The figure shows three views and two pictorial views of one solid part (mm, origin at its lowest corner). Answer the questions. Coordinates: 2 decimals unless noted, no trailing zeros. Write each loop counter-clockwise with the first axis right and the second up, starting at its lowest first coordinate (ties: lowest second). Pieces come first, ordered by that corner, then holes.
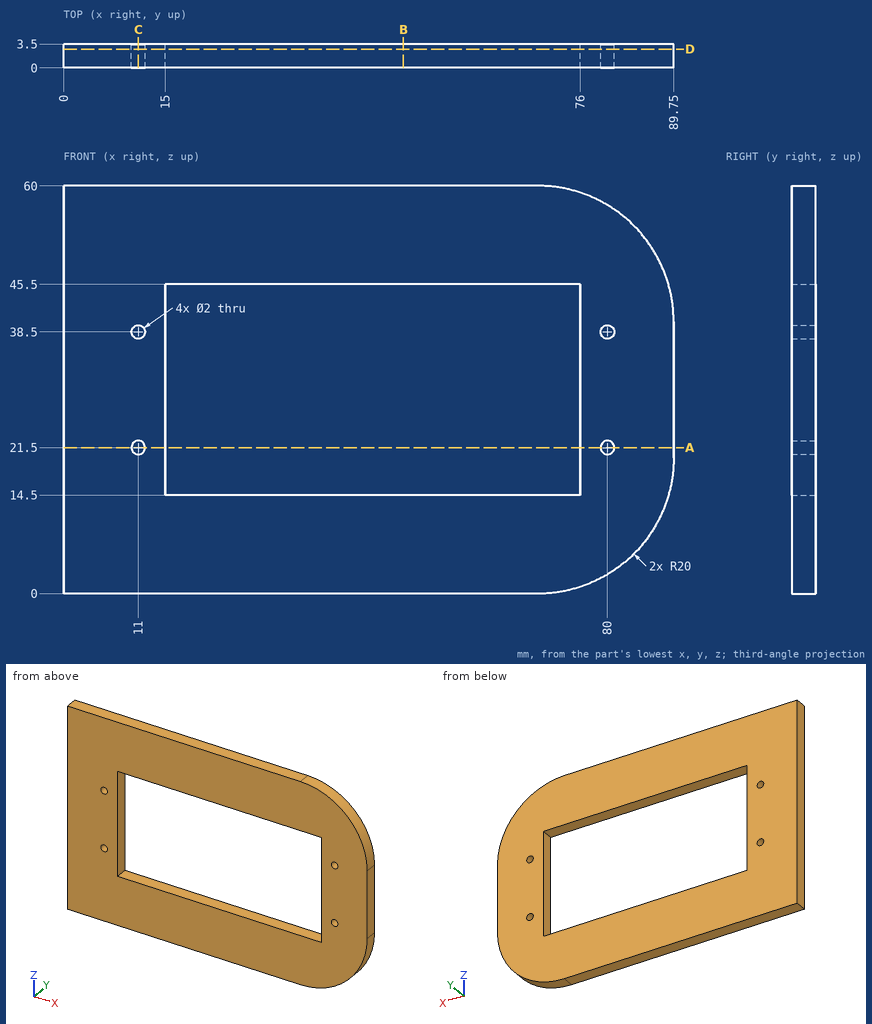
Q1. Find the intervals of material crossed by probe 1 along X at (y, z) = (1, 38.5); probe 2 along Z at (x, y) = (11, 1.35); probe 3 along Z at (x, y) = (51.5, 0.25), in increasing order.
Answers below:
probe 1: x = 0 to 10, 12 to 15, 76 to 79, 81 to 89.75
probe 2: z = 0 to 20.5, 22.5 to 37.5, 39.5 to 60
probe 3: z = 0 to 14.5, 45.5 to 60
Q2. The part is cut by section B-B, the plane x = 50. Write down the section's boundary in (y, z), then the cut area to 4 significant figures.
Answers below:
outline: (0, 0) - (3.5, 0) - (3.5, 14.5) - (0, 14.5) - close; (0, 45.5) - (3.5, 45.5) - (3.5, 60) - (0, 60) - close
area: 101.5 mm2
Q3. The part is cut by section D-D, the plane y = 2.75. Write down the section's boundary in (x, z).
Answers below:
outline: (0, 0) - (69.75, 0) arc R20 ccw to (89.75, 20) - (89.75, 40) arc R20 ccw to (69.75, 60) - (0, 60) - close; hole circle Ø2 at (11, 21.5); hole circle Ø2 at (11, 38.5); hole (15, 14.5) - (76, 14.5) - (76, 45.5) - (15, 45.5) - close; hole circle Ø2 at (80, 21.5); hole circle Ø2 at (80, 38.5)
Q4. The part is cut by section A-A, the plane z = 21.5. Write down the section's boundary in (x, y), then the cut area to 3 significant figures.
Answers below:
outline: (0, 0) - (10, 0) - (10, 3.5) - (0, 3.5) - close; (12, 0) - (15, 0) - (15, 3.5) - (12, 3.5) - close; (76, 0) - (79, 0) - (79, 3.5) - (76, 3.5) - close; (81, 0) - (89.75, 0) - (89.75, 3.5) - (81, 3.5) - close
area: 86.6 mm2
Q5. Given pin 1 (3 mm diameter, centred on x = 11, z = 38.5, fed in from +Y); pin 2 (1 mm diameter, centred on y = 1, z = 43, fed in from +X); pin 3 (2 mm diameter, centred on x = 71, y = 2, fed in from -Z), each flat-ended and moving along its own axis, determine where each tip first touches the part or whether it passes through.
Answers below:
pin 1: stops at y = 3.5
pin 2: stops at x = 89.59
pin 3: stops at z = 0
Q6. The part is cut by section C-C, the plane x = 11. Write down the section's boundary in (y, z), then the cut area to 3 significant figures.
Answers below:
outline: (0, 0) - (3.5, 0) - (3.5, 20.5) - (0, 20.5) - close; (0, 22.5) - (3.5, 22.5) - (3.5, 37.5) - (0, 37.5) - close; (0, 39.5) - (3.5, 39.5) - (3.5, 60) - (0, 60) - close
area: 196 mm2
